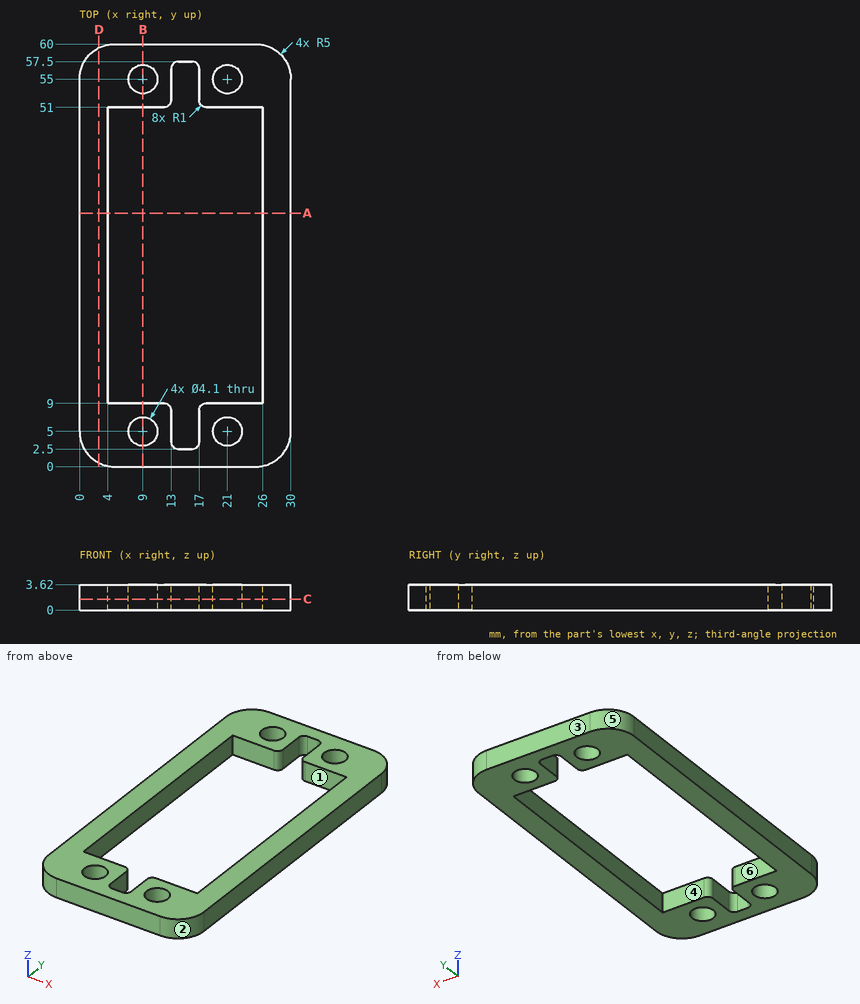
Answer from the drawing. Dimensions are ordinates in mm from the lowest x, y and z of the part. A direction names the side the tool comes from. Round coordinates to 2 decimals unless told otherwise and drop trailing zeros. Write each loop counter-clockwise with the first axis right and the second up, starting at its lowest first coordinate (ties: lowest second). Pieces come first, ordered by that corner, then holes. Notation, with made-up numbers: (-17.75, 23.5) - (35.25, 23.5) arc R11 ccw to (35.25, 33.5) - close; hole circle Ø1 at (54.25, -15). An arc over 180 degrees is marked (long way). One line per item, written item: value.
Q1. Find section A-A (y = 36). Determine the outline of the cut face in (x, z).
The answers:
outline: (0, 0) - (4, 0) - (4, 3.62) - (0, 3.62) - close; (26, 0) - (30, 0) - (30, 3.62) - (26, 3.62) - close
Q2. Find section B-B (x = 9). Determine the outline of the cut face in (y, z).
The answers:
outline: (0, 0) - (2.95, 0) - (2.95, 3.62) - (0, 3.62) - close; (7.05, 0) - (9, 0) - (9, 3.62) - (7.05, 3.62) - close; (51, 0) - (52.95, 0) - (52.95, 3.62) - (51, 3.62) - close; (57.05, 0) - (60, 0) - (60, 3.62) - (57.05, 3.62) - close
Q3. Which of the six approach directions +Z, -Z, +X, -X, +Y, -Y give full straight-line access (tool end or side, diameter ignored) to the marked faces 5 and 6?
The answers:
face 5: +Z, -Z, -X, +Y
face 6: +Z, -Z
Q4. This flat-tipped pin is pushed along its axis until it touches: P1, Ø1.5, axis at x = 24, y = 6.5, coming from the -Z side. Where does it stop, or does it pass through?
The answers:
P1: stops at z = 0
Q5. Find section D-D (x = 2.75). Determine the outline of the cut face in (y, z), and give its area (3 significant figures).
The answers:
outline: (0.53, 0) - (59.47, 0) - (59.47, 3.62) - (0.53, 3.62) - close
area: 213 mm2
Q6. Straight lines are drawn through the part: line 1 (Y direction, x = 9, z = 2.3); line 2 (X direction, y = 50, z = 0.35); line 3 (X direction, y = 8, z = 3.4). For each, find the intervals that lie inside material, in ascending order. Write a range as from..to.
The answers:
line 1: y = 0..2.95, 7.05..9, 51..52.95, 57.05..60
line 2: x = 0..4, 26..30
line 3: x = 0..13, 17..30
Q7. Find section C-C (z = 1.55). Count the separate pieces of the cut face and the enclosed holes in it, and give its area (3 significant figures).
The answers:
separate pieces: 1
enclosed holes: 5
area: 750 mm2
Q8. For a pull along Y with two mould halves and no side action, classify the marked faces 1, 2, 3 and 4 as pulls with the +Y half, pulls with the -Y half, needs draft (parallel to the pull), parting line crosses it, or undercut.
The answers:
face 1: undercut
face 2: pulls with the -Y half
face 3: pulls with the +Y half
face 4: undercut
